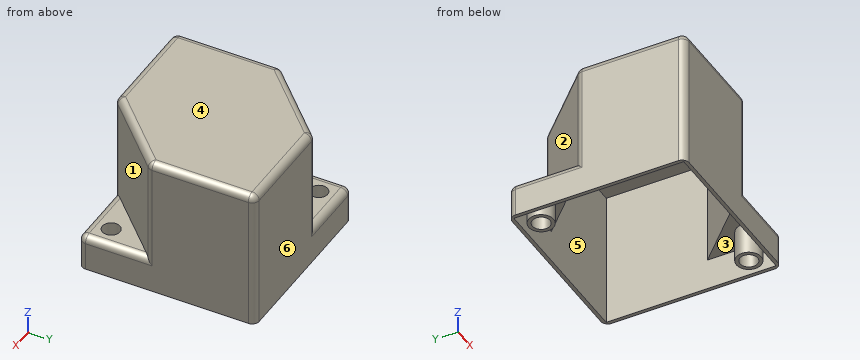
```python
from build123d import *

# Parameters (mm, degrees)
F0_W     = 127
F0_H     = 127
F1_DEPTH = 101.6
F3_DEPTH = 76.2
F4_R     = 6.35
F5_DEPTH = 203.2
F6_T     = -2.54
F7_R     = 5.08


# Not quite as in the source:
# - a feature names something its author has since deleted; it is built from what else it names


with BuildPart() as f1:
    # F0 (on Top) → F1 (new body)
    with BuildSketch(Plane.XY):
        with Locations((2.0048860461, 1.4262827701)):
            Rectangle(F0_W, F0_H)
    extrude(amount=F1_DEPTH)

    # F2 (on face) → F3 (cut)
    with BuildSketch(Plane.XY.offset(101.6)):
        Polygon((-61.4951139539, 14.1262827701), (-10.6951139539, 64.9262827701), (-61.4951139539, 64.9262827701), align=None)
        Polygon((65.5048860461, -62.0737172299), (65.5048860461, -11.2737172299), (14.7048860461, -62.0737172299), align=None)
    extrude(amount=-F3_DEPTH, mode=Mode.SUBTRACT)

    # F4 (on face) → F5 (cut)
    with BuildSketch(Plane.XY.offset(25.4)):
        with Locations((-46.2551139539, 49.6862827701)):
            Circle(F4_R)
        with Locations((50.2648860461, -46.8337172299)):
            Circle(F4_R)
    extrude(amount=-F5_DEPTH, mode=Mode.SUBTRACT)

    # F6
    f6_openings = [f1.faces().sort_by_distance(p)[0] for p in [
        (2.004886, 1.426283, 0),
    ]]
    offset(amount=F6_T, openings=f6_openings, kind=Kind.INTERSECTION)

    # F7
    f7_edges = [f1.edges().sort_by_distance(p)[0] for p in [
        (-36.095114, 39.526283, 101.6),
        (-61.495114, -23.973717, 101.6),
        (-23.395114, -62.073717, 101.6),
        (27.404886, 64.926283, 101.6),
        (65.504886, 26.826283, 101.6),
        (40.104886, -36.673717, 101.6),
        (-61.495114, 14.126283, 63.5),
        (-10.695114, 64.926283, 63.5),
        (-61.495114, 39.526283, 25.4),
        (-36.095114, 64.926283, 25.4),
        (-61.495114, 64.926283, 12.7),
        (-61.495114, -62.073717, 50.8),
        (14.704886, -62.073717, 63.5),
        (65.504886, -11.273717, 63.5),
        (65.504886, -36.673717, 25.4),
        (40.104886, -62.073717, 25.4),
        (65.504886, -62.073717, 12.7),
        (65.504886, 64.926283, 50.8),
    ]]
    fillet(f7_edges, radius=F7_R)


solid = f1.part
```
The listing builds one solid part. Answer for the finished solid, in the listing's coordinates (mm). Face numbers are marked on the shaded views. A direction names the side the tool comes from. Round coordinates to 2 decimals unless told otherwise and drop trailing zeros. Write each loop counter-clockwise with the first axis right and the second up, starting at its lowest first coordinate (ties: lowest second). Pieces come first, ordered by that corner, then holes. Notation, with made-up numbers: (45.5, 20) -> (104.5, 20) arc R19 cw to (104.5, 25) -> close; hole circle Ø4 at (76.25, 35.25). An arc over 180 degrees is marked (long way). Answer as a JSON object with one key per item and string values. Group by question number.
Q1. Section B-B (z = 16.5) is taken. Write down the section's boundary in (x, y), plus the area to 3 significant figures.
Q2. Each of these flat-tipped pins is pushed along its axis until it touches: pin 1 Ø10 at (x, y) = (14, -12.5) entering from -Z; pin 2 Ø16.5 at (x, y) = (50.26, -46.83) entering from -Z; pin 3 Ø5 at (y, z) = (-23.5, 72) entering from +X; pin 4 Ø15 at (x, y) = (29.5, -40) entering from -Z. Where does it stop, or does it pass through?
Q3. Section A-A (z = 94) is taken. Write down the section's boundary in (x, y).
Q4. Determine the mould class of the marked faces 4, 5 and 6 for opening direction Y: pulls with the +Y half, pulls with the -Y half, needs draft (parallel to the pull), parting line crosses it, or undercut.
Q5. Section C-C (x = -4.5) is taken. Write down the section's boundary in (y, z), plus the area to 3 significant figures.
Q6. Straight lines are drawn through the part: line 1 along Y through (x, z) = (0, 92); line 2 along X through (y, z) = (-4, 42); line 3 along Z through (x, y) = (20.5, 35). For each, find the intervals that lie inside material, in ascending order.
Q7. Which of the six approach directions +Z, -Z, +X, -X, +Y, -Y give full straight-line access (tool end or side, diameter ignored) to the marked faces 1, 2 and 3?
Check values:
{
 "1": {"outline": "(-61.5, -56.99) arc R5.08 ccw to (-56.42, -62.07) -> (60.42, -62.07) arc R5.08 ccw to (65.5, -56.99) -> (65.5, 59.85) arc R5.08 ccw to (60.42, 64.93) -> (-56.42, 64.93) arc R5.08 ccw to (-61.5, 59.85) -> close; circle Ø17.78 at (-46.26, 49.69); circle Ø17.78 at (50.26, -46.83); hole (-58.96, -59.53) -> (62.96, -59.53) -> (62.96, 62.39) -> (-58.96, 62.39) -> close; hole circle Ø12.7 at (-46.26, 49.69); hole circle Ø12.7 at (50.26, -46.83)", "area": "1,490 mm^2"},
 "2": {"pin 1": "z = 99.06", "pin 2": "z = 0", "pin 3": "x = 55.78", "pin 4": "z = 22.86"},
 "3": {"outline": "(-61.5, -56.99) arc R5.08 ccw to (-56.42, -62.07) -> (12.6, -62.07) arc R5.08 ccw to (16.19, -60.59) -> (64.02, -12.76) arc R5.08 ccw to (65.5, -9.17) -> (65.5, 59.85) arc R5.08 ccw to (60.42, 64.93) -> (-8.59, 64.93) arc R5.08 ccw to (-12.18, 63.44) -> (-60.01, 15.61) arc R5.08 ccw to (-61.5, 12.02) -> close; hole (-58.96, -59.53) -> (13.65, -59.53) -> (62.96, -10.22) -> (62.96, 62.39) -> (-9.64, 62.39) -> (-58.96, 13.07) -> close"},
 "4": {"face 4": "needs draft", "face 5": "undercut", "face 6": "pulls with the +Y half"},
 "5": {"outline": "(-62.07, 0) -> (-59.53, 0) -> (-59.53, 99.06) -> (62.39, 99.06) -> (62.39, 0) -> (64.93, 0) -> (64.93, 96.52) arc R5.08 ccw to (59.85, 101.6) -> (-56.99, 101.6) arc R5.08 ccw to (-62.07, 96.52) -> close", "area": "815 mm^2"},
 "6": {"line 1": "-62.07 to -59.53, 62.39 to 64.93", "line 2": "-61.5 to -58.96, 62.96 to 65.5", "line 3": "99.06 to 101.6"},
 "7": {"face 1": "+Z, +X, -Y", "face 2": "+Z, -X, +Y", "face 3": "-Z"}
}
